Check sheet for the drawn part. Datum: minimum x, y, z corner. Units: mm. Coordinates: 2 decimals unless noted, no trailing zeros. Order: outer loops, then holes, each group sorted by start corner. A loop starts at its lowest first (then second) coordinate and runs counter-clockwise, first axis right, second up. Notation, with made-up numbers: (12.5, 33) - (28.5, 33) arc R28 ccw to (28.5, 61) - close; hole circle Ø11 at (33.5, 89). An arc over 180 degrees is marked (long way). Put each result on its own line as item: value.
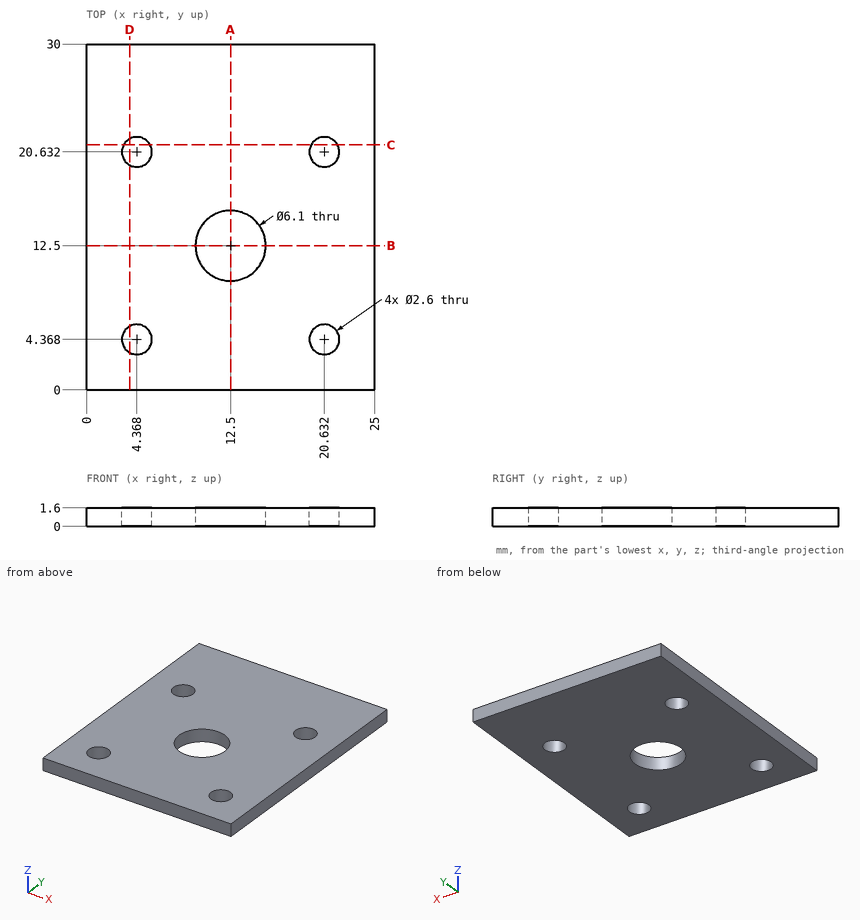
Q1. Section check B-B on y = 12.5. Record the boundary of the cut face in (x, z).
Answer block:
outline: (0, 0) - (9.45, 0) - (9.45, 1.6) - (0, 1.6) - close; (15.55, 0) - (25, 0) - (25, 1.6) - (15.55, 1.6) - close
Q2. Section check D-D on x = 3.75. Record the boundary of the cut face in (y, z) (1 decimal).
Answer block:
outline: (0, 0) - (3.2, 0) - (3.2, 1.6) - (0, 1.6) - close; (5.5, 0) - (19.5, 0) - (19.5, 1.6) - (5.5, 1.6) - close; (21.8, 0) - (30, 0) - (30, 1.6) - (21.8, 1.6) - close
Q3. Section check A-A on x = 12.5. Record the boundary of the cut face in (y, z).
Answer block:
outline: (0, 0) - (9.45, 0) - (9.45, 1.6) - (0, 1.6) - close; (15.55, 0) - (30, 0) - (30, 1.6) - (15.55, 1.6) - close
Q4. Thickness scan on L1, parallel to Y at x = 20.75, z = 0.2; L2, parallel to X at y = 20.75, z = 0.4; L3, parallel to Y at x = 5, z = 0.25 (1 decimal). Record the ranges inside material, lowest first. Write a range as [from, to].
Answer block:
L1: y = [0, 3.07], [5.66, 19.34], [21.93, 30]
L2: x = [0, 3.07], [5.66, 19.34], [21.93, 25]
L3: y = [0, 3.2], [5.5, 19.5], [21.8, 30]
Q5. Section check C-C on y = 21.25. Record the boundary of the cut face in (x, z) (1 decimal).
Answer block:
outline: (0, 0) - (3.2, 0) - (3.2, 1.6) - (0, 1.6) - close; (5.5, 0) - (19.5, 0) - (19.5, 1.6) - (5.5, 1.6) - close; (21.8, 0) - (25, 0) - (25, 1.6) - (21.8, 1.6) - close
